Source: CAD feature listing. Evaluate the final solid. Frame: model axes, mm. Face numbers are marked on the shaded views. A direction names the side the tool comes from. Coordinates: 2 decimals unless noted, no trailing zeros. Order: outer loops, then holes, each group sorted by start corner. A loop starts at its lowest first (then second) coordinate and runs counter-clockwise, first axis right, second up. Notation, with made-up numbers: (19.25, 10) -> (30.25, 10) arc R26 cw to (30.25, 47) -> close; hole circle Ø3 at (2.25, 25). An arc over 180 degrees is marked (long way). Put each result on its own line as item: value.
from build123d import *

# Parameters (mm, degrees)
BASPROSKE_W              = 10
BASPROSKE_H              = 12
TOOTHCUT_DEPTH           = 20.697716
TEETHCUTS_COUNT          = 14
TEETHCUTS_ANGLE          = 334.285714
BORSKE_R                 = 1.5
BORE_DEPTH               = 50.000051
BOSS_EXTRUDE1_DEPTH      = 10
BOSS_EXTRUDE2_START      = -40
BOSS_EXTRUDE2_DEPTH      = 40
CUT_EXTRUDE5_DEPTH       = 30
BOSS_EXTRUDE5_DEPTH      = 10
CHAMFER1_SIZE            = 10
BOSS_EXTRUDE6_DEPTH      = 3
BOSS_EXTRUDE6_DEPTH_BACK = 1
FILLET1_R                = 2
SKETCH12_R               = 3.15
CUT_EXTRUDE6_DEPTH       = 87.463865


with BuildPart() as part:
    # BasProSke → Base-Revolve (revolve)
    with BuildSketch(Plane(origin=(0, 0, 0), x_dir=(1, 0, 0), z_dir=(0, 1, 0)), mode=Mode.PRIVATE) as base_revolve_sk:
        with Locations((5, 6)):
            Rectangle(BASPROSKE_W, BASPROSKE_H)
    revolve(base_revolve_sk.sketch.rotate(Axis((-10, 0, 0), (1, 0, 0)), 180), axis=Axis((-10, 0, 0), (1, 0, 0)))

    # TooCutSke → ToothCut (cut, through all)
    with BuildSketch(Plane(origin=(0, 0, 0), x_dir=(0, 0, -1), z_dir=(1, 0, 0))):
        with BuildLine():
            ThreePointArc((0.804846, 8.586361), (0, 8.624), (-0.804846, 8.586361))
            ThreePointArc((-0.804846, 8.586361), (-1.237812, 10.362618), (-2.384428, 11.786634))
            ThreePointArc((-2.384428, 11.786634), (0, 12.0254), (2.384428, 11.786634))
            ThreePointArc((2.384428, 11.786634), (1.237812, 10.362618), (0.804846, 8.586361))
        make_face()
    toothcut = extrude(amount=TOOTHCUT_DEPTH, mode=Mode.SUBTRACT)

    # TeethCuts: ToothCut ×14 about axis
    teethcuts_axis = Axis((-10, 0, 0), (1, 0, 0))
    for i in range(1, TEETHCUTS_COUNT):
        add(toothcut.rotate(teethcuts_axis, i * TEETHCUTS_ANGLE / (TEETHCUTS_COUNT - 1)), mode=Mode.SUBTRACT)

    # BorSke → Bore (cut, symmetric)
    with BuildSketch(Plane(origin=(0, 0, 0), x_dir=(0, 0, -1), z_dir=(1, 0, 0))):
        with Locations(Location((0, 0, 0), (0, 0, 180))):
            Circle(BORSKE_R)
    extrude(amount=BORE_DEPTH, both=True, mode=Mode.SUBTRACT)

    # Sketch1 → Boss-Extrude1 (add)
    with BuildSketch(Plane(origin=(10, 0, 0), x_dir=(0, 0, -1), z_dir=(1, 0, 0))):
        with BuildLine():
            Line((0, 29), (0, 4))
            Line((0, 4), (8, 4))
            Line((8, 4), (20, 29))
            Line((20, 29), (20, 64))
            Line((20, 64), (0, 74))
            Line((0, 74), (0, 64))
            ThreePointArc((0, 64), (9.391813, 46.5), (0, 29))
        make_face()
    extrude(amount=-BOSS_EXTRUDE1_DEPTH)

    # Sketch2 → Boss-Extrude2 (add)
    with BuildSketch(Plane.ZY.offset(BOSS_EXTRUDE2_START)):
        with BuildLine():
            Line((-20, 29), (-7.698792, 3.139406))
            Line((-7.698792, 3.139406), (0, 8.624))
            Line((0, 8.624), (0, 29))
            ThreePointArc((0, 29), (-9.391813, 46.5), (0, 64))
            Line((0, 64), (0, 74))
            Line((0, 74), (-20, 64))
            Line((-20, 64), (-20, 29))
        make_face()
    extrude(amount=BOSS_EXTRUDE2_DEPTH)

    # Sketch9 → Cut-Extrude5 (cut)
    with BuildSketch(Plane(origin=(40, 0, 0), x_dir=(0, 0, -1), z_dir=(1, 0, 0))):
        Polygon((7.698792, 3.139406), (0, 8.624), (0, 18.812), (13.849396, 16.069703), align=None)
    extrude(amount=-CUT_EXTRUDE5_DEPTH, mode=Mode.SUBTRACT)

    # Sketch10 → Boss-Extrude5 (add)
    with BuildSketch(Plane(origin=(10, 0, 0), x_dir=(0, 0, -1), z_dir=(1, 0, 0))):
        Polygon((0, 18.812), (0, 10.812), (11.330599, 10.774484), (15.153835, 18.812), align=None)
    extrude(amount=BOSS_EXTRUDE5_DEPTH)

    # Chamfer1
    # the kernel refuses this chamfer: 10 mm, written as the material it takes off along each edge
    with BuildSketch(Plane(origin=(20, 10.897149, 25.716689), x_dir=(0.027495876610586313, 0.9996164375424699, -0.003309768015556128), z_dir=(0, -0.0033110198561701067, -0.999994518558733))) as chamfer1_piece_1_section:
        Polygon((CHAMFER1_SIZE * 0.999621916911, -CHAMFER1_SIZE * 0.0274958766106), (-CHAMFER1_SIZE * 0.0274958766106, -CHAMFER1_SIZE * 0.999621916911), (0, 0), align=None)
    chamfer1_piece_1 = extrude(amount=62.764321, mode=Mode.PRIVATE)
    chamfer1_piece_1 = split(chamfer1_piece_1, bisect_by=Plane(origin=(16.383831, 18.515288, -1.498481), z_dir=(0, -0.980954576947178, 0.19423727234077168)), keep=Keep.TOP, mode=Mode.PRIVATE)
    chamfer1_piece_1 = split(chamfer1_piece_1, bisect_by=Plane(origin=(10, 13.486301, -0.502699), z_dir=(1, 0, 0)), keep=Keep.TOP, mode=Mode.PRIVATE)
    add(chamfer1_piece_1, mode=Mode.SUBTRACT)

    # Sketch11 → Boss-Extrude6 (add, two sides: drawn at the far end of the back side and taken through both)
    with BuildSketch(Plane(origin=(10, 0, 0), x_dir=(0, 0, -1), z_dir=(1, 0, 0)).offset(-BOSS_EXTRUDE6_DEPTH_BACK)):
        with BuildLine():
            Line((-2.358667, 11.765912), (-1.230525, 10.347781))
            Line((-1.230525, 10.347781), (-0.81596, 8.618917))
            ThreePointArc((-0.81596, 8.618917), (-3.657356, -7.846992), (7.125155, 4.917692))
            Line((7.125155, 4.917692), (8.811802, 5.479265))
            Line((8.811802, 5.479265), (10.669566, 5.491846))
            ThreePointArc((10.669566, 5.491846), (-5.206605, -10.811626), (-2.358667, 11.765912))
        make_face()
    extrude(amount=BOSS_EXTRUDE6_DEPTH + BOSS_EXTRUDE6_DEPTH_BACK)

    # Fillet1
    fillet1_edges = [part.edges().sort_by_distance(p)[0] for p in [
        (13, -10.811626, 5.206605),
    ]]
    fillet(fillet1_edges, radius=FILLET1_R)

    # Sketch12 → Cut-Extrude6 (cut, through all)
    with BuildSketch(Plane.ZY):
        Circle(SKETCH12_R)
    extrude(amount=-CUT_EXTRUDE6_DEPTH, mode=Mode.SUBTRACT)


solid = part.part
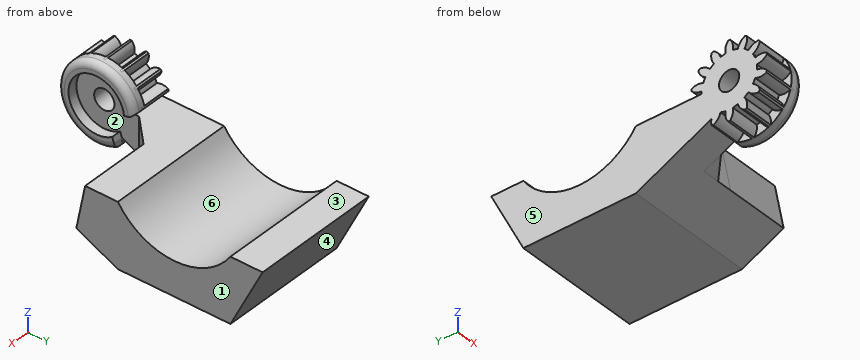
1. Cut plane B-B on y = 26.5. Output: boundary loops of the cut face in (x, z).
Numbers:
outline: (0, -18.81) -> (40, -18.81) -> (40, 0) -> (0, 0) -> close
2. Pull-direction query (Y, two-part tool) for the marked faces 4, 5 and 6; classes: pulls with the +Y half, pulls with the -Y half, needs draft (parallel to the pull), parting line crosses it, or undercut.
Numbers:
face 4: pulls with the +Y half
face 5: needs draft
face 6: undercut
3. First-contact query: pin 1 (1.1 mm diameter, centred on y = -2.5, z = -10, fed in from -X); pin 2 (3 mm diameter, centred on y = 2.5, z = -15, fed in from +X); pin 3 (4 mm diameter, centred on x = 25.5, z = -8, fed in from +Y); pin 4 (1 mm diameter, centred on x = 27.5, z = -14.5, fed in from +Y). Flat tips, straight axial feed; report the tip coordinate or a pass-through.
Numbers:
pin 1: stops at x = 9
pin 2: passes through
pin 3: stops at y = 71
pin 4: stops at y = 67
4. Set-up query: the marked faces 1, 2 and 3. Return all of +Z, -Z, +X, -X, +Y, -Y with unobstructed straight access to the full face (end or side cutting, diameter ignored); none if empty.
Numbers:
face 1: +Z, -Z, +X, +Y, -Y
face 2: +X
face 3: +Z, +X, -X, +Y
5. Ray query, line 1 along X through (y, z) = (8, 4.5); line 2 along X through (y, z) = (-2, 7); line 3 along Z through (x, y) = (11, 0). Return the intervals inside material, ascending.
Numbers:
line 1: x = 9 to 13
line 2: x = 0 to 10
line 3: z = -12 to -8.66, 8.66 to 12
6. Cut plane D-D on y = 46. Output: boundary loops of the cut face in (x, z), plus the area to 3 significant figures.
Numbers:
outline: (0, -20) -> (40, -20) -> (40, -9.39) -> (0, -9.39) -> close
area: 425 mm2
7. Cut plane A-A on x = 25.5. Output: boundary loops of the cut face in (y, z).
Numbers:
outline: (16.07, -13.85) -> (29, -20) -> (64, -20) -> (74, 0) -> (64, 0) arc R21 cw to (29, 0) -> (18.81, 0) -> close
8. Cut plane C-C on x = 14. Output: boundary loops of the cut face in (y, z).
Numbers:
outline: (14.77, -13.23) -> (29, -20) -> (64, -20) -> (74, 0) -> (64, 0) arc R21 cw to (29, 0) -> (14.81, 0) -> close
